```python
from build123d import *

# Parameters (mm, degrees)
AUFSATZ_LINEAR_AUSTRAGEN1_DEPTH = 10
VERRUNDUNG1_R                   = 1
SKIZZE2_R                       = 1.6
SCHNITT_LINEAR_AUSTRAGEN1_DEPTH = 10
SKIZZE3_R                       = 3.15
SCHNITT_LINEAR_AUSTRAGEN2_DEPTH = 20


with BuildPart() as part:
    # Skizze1 → Aufsatz-Linear austragen1 (new body)
    with BuildSketch(Plane.XY):
        with BuildLine():
            Line((-34.551329334, 20.352288355), (-44.718553427, 26.341241038))
            ThreePointArc((-44.718553427, 26.341241038), (0, 51.9), (44.718553427, 26.341241038))
            Line((44.718553427, 26.341241038), (34.551329334, 20.352288355))
            ThreePointArc((34.551329334, 20.352288355), (0, 40.1), (-34.551329334, 20.352288355))
        make_face()
    extrude(amount=AUFSATZ_LINEAR_AUSTRAGEN1_DEPTH)

    # Verrundung1
    verrundung1_edges = [part.edges().sort_by_distance(p)[0] for p in [
        (-34.551329334, 20.352288355, 5),
        (-44.718553427, 26.341241038, 5),
        (44.718553427, 26.341241038, 5),
        (34.551329334, 20.352288355, 5),
    ]]
    fillet(verrundung1_edges, radius=VERRUNDUNG1_R)

    # Skizze2 → Schnitt-Linear austragen1 (cut)
    with BuildSketch(Plane.XY.offset(10)):
        with Locations((0, 46)):
            Circle(SKIZZE2_R)
        with Locations((35.964248194, 28.680530886)):
            Circle(SKIZZE2_R)
        with Locations((-35.964248194, 28.680530886)):
            Circle(SKIZZE2_R)
    extrude(amount=-SCHNITT_LINEAR_AUSTRAGEN1_DEPTH, mode=Mode.SUBTRACT)

    # Skizze3 → Schnitt-Linear austragen2 (cut)
    with BuildSketch(Plane(origin=(0, 51.9, 0), x_dir=(1, 0, 0), z_dir=(0, 1, 0))):
        with Locations(Location((-35, -5, 0), (0, 0, 270))):
            Circle(SKIZZE3_R)
        with Locations(Location((35, -5, 0), (0, 0, 270))):
            Circle(SKIZZE3_R)
    extrude(amount=-SCHNITT_LINEAR_AUSTRAGEN2_DEPTH, mode=Mode.SUBTRACT)


solid = part.part
```
CAD build for the part. Positions are in the model's coordinates, mm. A direction names the side the tool comes from. Coordinates: 2 decimals unless noted, no trailing zeros. Order: outer loops, then holes, each group sorted by start corner. A loop starts at its lowest first (then second) coordinate and runs counter-clockwise, first axis right, second up. Notation, with made-up numbers: M 1.5,76 L 39.5,76 A19 ccw 39.5,103 Z; hole C 41,11 d6. An arc over 180 degrees is marked long. Answer as CSV lines item,"result".
1) Cut at B-B (y = 33.5). List the corners of the cut face in (x, z).
Verdict:
outline,"M -39.64,0 L -22.04,0 L -22.04,10 L -39.64,10 Z; M 22.04,0 L 39.64,0 L 39.64,10 L 22.04,10 Z; hole C -35,5 d6.3; hole C 35,5 d6.3"
2) Cut at A-A (x = 0). List the corners of the cut face in (y, z), then the cut area to 3 significant figures.
Verdict:
outline,"M 40.1,0 L 44.4,0 L 44.4,10 L 40.1,10 Z; M 47.6,0 L 51.9,0 L 51.9,10 L 47.6,10 Z"
area,"86.0 mm2"
3) Cut at D-D (x = 22). List the corners of the cut face in (y, z), then the cut area to 3 significant figures.
Verdict:
outline,"M 33.53,0 L 47.01,0 L 47.01,10 L 33.53,10 Z"
area,"135 mm2"
4) Flat gauge pins, fed straight in: P1, Ø4, axis at x = -28, z = 5.5, coming from the -Y side; P2, Ø5, axis at x = 34.5, z = 4, coming from the +Y side; P3, Ø1.9, axis at x = -35.5, z = 5.5, coming from the +Y side. Where does each tip first touch, or does it go through?
Verdict:
P1,"y = 26.61"
P2,"y = 40.86"
P3,"y = 31.9"
5) 3-axis set-ups, long thin cutter, end or side, ignore diameter. For faces 4 (the flat face through (39.685, 23.376, 4.93)), 5 (the flat face through (-35, 31.9, 5)): which of +Z, -Z, +X, -X, +Y, -Y reach the whole face in a straight line?
Verdict:
face 4,"+Z, -Z, +X, -Y"
face 5,"+Y"
6) Cut at C-C (y = 46). List the corners of the cut face in (x, z).
Verdict:
outline,"M -24.03,0 L -1.6,0 L -1.6,10 L -24.03,10 Z; M 1.6,0 L 24.03,0 L 24.03,10 L 1.6,10 Z"
7) Drill centre lines: L1, parallel to Z at x = -35, y = 37; L2, parallel to X at y = 33, z = 5.75; L3, parallel to X at y = 36, z = 5. Where is each one in solid material? Low to high. Write a range as from..to.
Verdict:
L1,"0..1.85, 8.15..10"
L2,"-40.06..-38.06, -31.94..-22.78, 22.78..31.94, 38.06..40.06"
L3,"-31.85..-17.66, 17.66..31.85"
8) Mould opens along X. For faces 1 (the flat face through (-39.57, 23.31, 4.93)), 2 (the cylindrical face through (-0.74, 51.895, 4.93)), 3 (the cylindrical face through (-31.877, 35.494, 4.59)) say: released by +X, released by -X, zero draft, split by the parting line, or undercut.
Verdict:
face 1,"released by -X"
face 2,"split by the parting line"
face 3,"undercut"
